Design review of the part shown in the three views and the two pictorial views. Dimensions are in mm from the part's minimum x, y and z. A direction names the side the tool comes from. Round coordinates to 2 decimals unless told otherwise and drop trailing zeros. Order: outer loops, then holes, each group sorted by start corner. A loop starts at its lowest first (then second) coordinate and runs counter-clockwise, first axis right, second up. Notation, with made-up numbers: (-36, -28.5) - (7, -28.5) arc R7 cw to (7, -17.5) - close; hole circle Ø7 at (85, -26). An arc over 180 degrees is marked (long way). One line per item, written item: value.
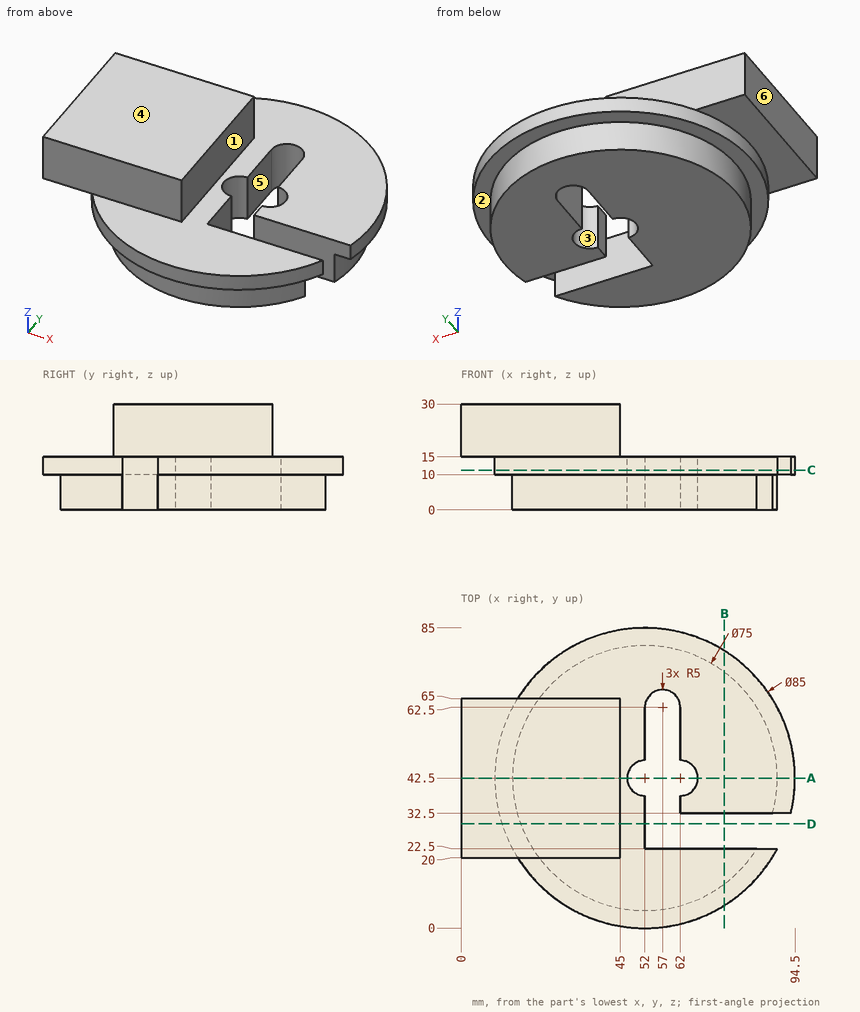
Item 1: Take a section at A-A (y = 42.5). Write out the cut boundary in (x, z).
Returned:
outline: (0, 15) - (9.5, 15) - (9.5, 10) - (14.5, 10) - (14.5, 0) - (47, 0) - (47, 15) - (45, 15) - (45, 30) - (0, 30) - close; (67, 0) - (89.5, 0) - (89.5, 10) - (94.5, 10) - (94.5, 15) - (67, 15) - close
Item 2: Take a section at C-C (z = 11.25). Write out the cut boundary in (x, y), plus the area to 3 significant figures.
Returned:
outline: (52, 22.5) - (52, 37.5) arc R5 cw to (52, 47.5) - (52, 62.5) arc R5 cw to (62, 62.5) - (62, 47.5) arc R5 cw to (62, 37.5) - (62, 32.5) - (93.31, 32.5) arc R42.5 ccw (long way) to (89.5, 22.5) - close
area: 4,860 mm^2
Item 3: Wall thickness on line 1 (Z direction, x = 81, y = 22); line 2 (X direction, y = 45, z = 17); line 3 (Y direction, x = 11, z = 16): over which ranges is each line inside the solid? List them lowest first.
Returned:
line 1: 0 to 15
line 2: 0 to 45
line 3: 20 to 65
Item 4: The part is to be moulded in two halves that separate along X. For the marked faces 4, 5 and 6, say which applies: +X half, -X half, draft (parallel to the pull), parting line (faces both ways), or undercut.
Returned:
face 4: draft
face 5: undercut
face 6: -X half
Item 5: Take a section at D-D (y = 29.5). Write out the cut boundary in (x, z), plus the area to 3 significant figures.
Returned:
outline: (0, 15) - (11.54, 15) - (11.54, 10) - (16.83, 10) - (16.83, 0) - (52, 0) - (52, 15) - (45, 15) - (45, 30) - (0, 30) - close
area: 1,230 mm^2
Item 6: Take a section at B-B (x = 74.5). Write out the cut boundary in (y, z).
Returned:
outline: (6.44, 10) - (12.5, 10) - (12.5, 0) - (22.5, 0) - (22.5, 15) - (6.44, 15) - close; (32.5, 0) - (72.5, 0) - (72.5, 10) - (78.56, 10) - (78.56, 15) - (32.5, 15) - close
Item 7: For P1, Ø2, axis at y = 23.5, z = 24, coming from the +X side; P2, Ø16.5, axis at x = 33, z = 19, coming from the -Y side; P3, Ø2, axis at y = 31.5, z = 17, coming from the -X side; P4, Ø4, axis at x = 84.5, z = 10.5, coming from the -Y side, all flat-tipped, find the tip position at first contact; note any pin that passes through.
Returned:
P1: x = 45
P2: y = 1.67
P3: x = 0
P4: y = 12.9
Item 8: Machinability: for the marked faces 1, 2 and 3, which of the approach directions +Z, -Z, +X, -X, +Y, -Y give a long, thin tool a straight path to every point of the face, cutting with its end or side? Answer none if there is none.
Returned:
face 1: +Z, +X, +Y, -Y
face 2: -Z
face 3: +Z, -Z
